Check sheet for the modelled part. Datum: model origin and axes. Units: mm. A direction names the side the tool comes from. Coordinates: 2 decimals unless noted, no trailing zeros. Loops run counter-clockwise (first coordinate to the right, second up) from the corner with the lowest first, then second, coordinate; pieces in that order, holes last. Notation, with made-up numbers: M 60.25,-33.75 L 81.25,-33.75 A38 ccw 81.25,5.25 Z; hole C 16.25,-34.75 d1. An arc over 180 degrees is marked long. Write each question's results on one line, items separated by ' | '. Start each with the question number.
from build123d import *

# Parameters (mm, degrees)
SKETCH1_W           = 38.1
SKETCH1_H           = 19.05
SKETCH1_W_2         = 31.75
SKETCH1_H_2         = 12.7
BOSS_EXTRUDE1_DEPTH = 133.35
SKETCH2_R           = 3.175
CUT_EXTRUDE1_DEPTH  = 39.1
SKETCH3_R           = 2.0193
CUT_EXTRUDE2_DEPTH  = 39.1
CUT_EXTRUDE3_REACH  = 5.175
SKETCH4_R           = 4.7625
SKETCH5_R           = 2.54
CUT_EXTRUDE4_DEPTH  = 20.05


with BuildPart() as part:
    # Sketch1 → Boss-Extrude1 (new body)
    with BuildSketch(Plane(origin=(0, 0, 0), x_dir=(1, 0, 0), z_dir=(0, 1, 0))):
        with Locations((19.05, 9.525)):
            Rectangle(SKETCH1_W, SKETCH1_H)
        with Locations((19.05, 9.525)):
            Rectangle(SKETCH1_W_2, SKETCH1_H_2, mode=Mode.SUBTRACT)
    extrude(amount=BOSS_EXTRUDE1_DEPTH)

    # Sketch2 → Cut-Extrude1 (cut, through all)
    with BuildSketch(Plane(origin=(38.1, 0, 0), x_dir=(0, 0, -1), z_dir=(1, 0, 0))):
        with Locations((9.525, 95.25)):
            Circle(SKETCH2_R)
        with Locations((9.525, 120.65)):
            Circle(SKETCH2_R)
    extrude(amount=-CUT_EXTRUDE1_DEPTH, mode=Mode.SUBTRACT)

    # Sketch3 → Cut-Extrude2 (cut, through all)
    with BuildSketch(Plane.ZY):
        with Locations((-8.8564, 19.789753907)):
            Circle(SKETCH3_R)
        with Locations((-8.8564, 45.189753907)):
            Circle(SKETCH3_R)
    extrude(amount=-CUT_EXTRUDE2_DEPTH, mode=Mode.SUBTRACT)

    # Sketch4 → Cut-Extrude3 (cut, up to next)
    with BuildSketch(Plane.ZY.offset(-34.925), mode=Mode.PRIVATE) as cut_extrude3_sk1:
        with Locations((-8.8564, 45.189753907)):
            Circle(SKETCH4_R)
    cut_extrude3_tool1 = extrude(cut_extrude3_sk1.sketch, amount=-CUT_EXTRUDE3_REACH, mode=Mode.PRIVATE) & part.part
    add(cut_extrude3_tool1.solids().sort_by_distance((34.925, 45.189754, -8.8564))[0], mode=Mode.SUBTRACT)
    # Sketch4 → Cut-Extrude3 (cut, up to next)
    with BuildSketch(Plane.ZY.offset(-34.925), mode=Mode.PRIVATE) as cut_extrude3_sk2:
        with Locations((-8.8564, 19.789753907)):
            Circle(SKETCH4_R)
    cut_extrude3_tool2 = extrude(cut_extrude3_sk2.sketch, amount=-CUT_EXTRUDE3_REACH, mode=Mode.PRIVATE) & part.part
    add(cut_extrude3_tool2.solids().sort_by_distance((34.925, 19.789754, -8.8564))[0], mode=Mode.SUBTRACT)

    # Sketch5 → Cut-Extrude4 (cut, through all)
    with BuildSketch(Plane(origin=(0, 0, -19.05), x_dir=(-1, 0, 0), z_dir=(0, 0, -1))):
        with Locations((-19.272235529, 69.491227214)):
            Circle(SKETCH5_R)
        with Locations((-19.272235529, 110.945613607)):
            Circle(SKETCH5_R)
    extrude(amount=-CUT_EXTRUDE4_DEPTH, mode=Mode.SUBTRACT)


solid = part.part
1) Thickness scan on probe 1 along X at (y, z) = (64.5, -8) (3 decimals); probe 2 along Z at (x, y) = (5.5, 64.5) (3 decimals); probe 3 along Z at (x, y) = (37, 95). Record the ranges inside material, lowest first.
2) Set-up check for faces 4 (the cylindrical face through (1.6, 44.4, -7)), 5 (the flat face through (34.925, 66, -9)), 6 (the cylindrical face through (36, 49, -6)): record each of +Z, -Z, +X, -X, +Y, -Y from which the full face is reachable in a straight line by a thin tool's end or side.
3) Section check C-C (x = 19). Enter the section's corners in (y, z) (3 decimals).
4) Section check A-A (y = 95.25). Enter the section's corners in (x, z) (3 decimals), then the cut area to 3 significant figures.
5) Release check for a two-part mould opening along Y. For faces 1 (the flat face through (3.175, 66, -9)), 2 (the cylindrical face through (19.823, 108.466, -17.485)), 3 (the flat face through (19, 0, -18)) record: +Y half, -Y half, draft (parallel to the pull), parting line (faces both ways), or undercut.
6) Section check B-B (x = 25). Enter the section's corners in (y, z) (3 decimals).
7) Gauge pin test, flat end, axial feed: P1, Ø8, axis at y = 109.5, z = -15.5, coming from the -X side. Record the tip position at first contact, or that the pin passes through.
Return value:
1) probe 1: x = 0 to 3.175, 34.925 to 38.1 | probe 2: z = -19.05 to -15.875, -3.175 to 0 | probe 3: z = -19.05 to -12.69, -6.36 to 0
2) face 4: +X, -X | face 5: +Y, -Y | face 6: +X
3) outline: M 0,-19.05 L 66.966,-19.05 L 66.966,-15.875 L 0,-15.875 Z; M 0,-3.175 L 66.966,-3.175 L 66.966,0 L 0,0 Z; M 72.017,-19.05 L 108.42,-19.05 L 108.42,-15.875 L 72.017,-15.875 Z; M 72.017,-3.175 L 108.42,-3.175 L 108.42,0 L 72.017,0 Z; M 113.471,-19.05 L 133.35,-19.05 L 133.35,-15.875 L 113.471,-15.875 Z; M 113.471,-3.175 L 133.35,-3.175 L 133.35,0 L 113.471,0 Z
4) outline: M 0,-19.05 L 38.1,-19.05 L 38.1,-12.7 L 34.925,-12.7 L 34.925,-15.875 L 3.175,-15.875 L 3.175,-12.7 L 0,-12.7 Z; M 0,-6.35 L 3.175,-6.35 L 3.175,-3.175 L 34.925,-3.175 L 34.925,-6.35 L 38.1,-6.35 L 38.1,0 L 0,0 Z | area: 282 mm2
5) face 1: draft | face 2: undercut | face 3: -Y half
6) outline: M 0,-19.05 L 133.35,-19.05 L 133.35,-15.875 L 0,-15.875 Z; M 0,-3.175 L 133.35,-3.175 L 133.35,0 L 0,0 Z
7) P1: stops at x = 0
